Autodesk Fusion 360 part; units mm, degrees
sketch "Back Panel" plane through (0, 0, 0) normal (1, 0, 0) x (0, 1, 0)
  line L0 (0, 0) -> (6, 0)
  line L1 (6, 0) -> (6, 500.8)
  line L2 (0, 500.8) -> (0, 0)
  line L3 (0, 500.8) -> (0, 503.263)
  line L4 (6, 500.8) -> (0, 503.263)
  dimension "d8" = 6
  dimension "d9" = 500.8
  dimension "d10" = 2.463
  dimension "d11" = 112.318
extrude "Extrude2" add sketch "Back Panel" along normal blind 270
sketch "Switch Hole" plane through (0, 6, 0) normal (0, 1, 0) x (-1, 0, 0)
  line L0 (0, 0) -> (0, 500.8)
  line L1 (0, 500.8) -> (-270, 500.8)
  line L2 (-270, 500.8) -> (-270, 0)
  line L3 (-270, 0) -> (0, 0)
  line L4 (-234, 37) -> (-215, 37)
  line L5 (-215, 37) -> (-215, 24)
  line L6 (-215, 24) -> (-234, 24)
  line L7 (-234, 24) -> (-234, 37)
  dimension "d14" = 19
  dimension "d15" = 13
  dimension "d16" = 36
  dimension "d17" = 24
extrude "Extrude3" cut sketch "Switch Hole" against normal blind 6 contours L4 L5 L6 L7
sketch "Bottom Access Panel" plane through (0, 6, 0) normal (0, 1, 0) x (-1, 0, 0)
  line L0 (-215, 37) -> (-215, 24)
  line L1 (-215, 24) -> (-234, 24)
  line L2 (-234, 24) -> (-234, 37)
  line L3 (-234, 37) -> (-215, 37)
  line L4 (0, 0) -> (0, 500.8)
  line L5 (0, 500.8) -> (-270, 500.8)
  line L6 (-270, 500.8) -> (-270, 0)
  line L7 (-270, 0) -> (0, 0)
  line L8 (-205, 188) -> (-65, 188)
  line L9 (-65, 188) -> (-65, 48)
  line L10 (-65, 48) -> (-205, 48)
  line L11 (-205, 48) -> (-205, 188)
  dimension "d20" = 48
  dimension "d21" = 65
  dimension "d22" = 65
  dimension "d28" = 140
  dimension "d29" = 140
  dimension "d30" = 24
  dimension "d31" = 11
  dimension "d32" = 13
  dimension "d33" = 188
extrude "Extrude4" cut sketch "Bottom Access Panel" against normal blind 6 contours L8 L9 L10 L11
fillet "Fillet1" radius 8 4 edges at (65, 3, 188) (65, 3, 48) (205, 3, 48) (205, 3, 188)
sketch "Top Access Panel" plane through (0, 6, 0) normal (0, 1, 0) x (-1, 0, 0)
  line L0 (-65, 180) -> (-65, 56)
  arc A0 (-73, 48) -> (-65, 56) centre (-73, 56) ccw
  line L1 (-73, 48) -> (-197, 48)
  arc A1 (-205, 56) -> (-197, 48) centre (-197, 56) ccw
  line L2 (-205, 56) -> (-205, 180)
  arc A2 (-197, 188) -> (-205, 180) centre (-197, 180) ccw
  line L3 (-197, 188) -> (-73, 188)
  arc A3 (-65, 180) -> (-73, 188) centre (-73, 180) ccw
  line L4 (-215, 37) -> (-215, 24)
  line L5 (-215, 24) -> (-234, 24)
  line L6 (-234, 24) -> (-234, 37)
  line L7 (-234, 37) -> (-215, 37)
  line L8 (0, 0) -> (0, 500.8)
  line L9 (0, 500.8) -> (-270, 500.8)
  line L10 (-270, 500.8) -> (-270, 0)
  line L11 (-270, 0) -> (0, 0)
  line L12 (-195, 473.263) -> (-75, 473.263)
  line L13 (-75, 473.263) -> (-75, 383.263)
  line L14 (-75, 383.263) -> (-195, 383.263)
  line L15 (-195, 383.263) -> (-195, 473.263)
  line L16 (-180, 473.263) -> (-90, 473.263)
  line L17 (0, 503.263) -> (-270, 503.263)
  dimension "d34" = 120
  dimension "d35" = 140
  dimension "d36" = 75
  dimension "d37" = 75
  dimension "d38" = 65
  dimension "d39" = 65
  dimension "d45" = 90
  dimension "d49" = 30
extrude "Extrude5" cut sketch "Top Access Panel" against normal blind 6 contours L12 L13 L14 L15 L16
fillet "Fillet2" radius 8 4 edges at (75, 3, 473.263) (195, 3, 473.263) (195, 3, 383.263) (75, 3, 383.263)
equation "MDFThickness = 6 mm"
equation "d16 = ( 18 * 2 ) * 1 mm"
equation "d17 = ( 12 * 2 ) * 1 mm"
equation "filletRadius = 8 mm"
equation "d27 = filletRadius"
equation "d36 = ( ( 270 - 120 ) / 2 ) * 1 mm"
equation "d54 = filletRadius"
CAD build for the part. Positions are in the model's coordinates, mm. Round coordinates to 2 decimals unless told otherwise and drop trailing zeros. Loops run counter-clockwise (first coordinate to the right, second up) from the corner with the lowest first, then second, coordinate; pieces in that order, holes last. Notation, with made-up numbers: M -5.75,71.25 L 29.25,71.25 A22 cw 29.25,99.25 Z; hole C 1,86.5 d11. An arc over 180 degrees is marked long. One line per question, with ' | ' between items. Start each with the question number.
Item 1: Cut at B-B, the plane z = 115.5. Write the cut outline in (x, y).
Item 2: Cut at C-C, the plane y = 1.25. Write the cut outline in (x, z).
Item 3: Cut at D-D, the plane z = 422. Write the cut outline in (x, y), plus the area to 3 significant figures.
Item 4: Wall check: line 1 (Z direction, x = 168, y = 2.35); line 2 (Z direction, x = 76, y = 4.1); line 3 (X direction, y = 2.45, z = 61.5). Give the ranges that are in metal, low to high.
Item 5: Pin check, flat tips, straight feed: pin 1 Ø1.8 at (x, y) = (220.5, 2.5) entering from +Z; pin 2 Ø3 at (x, y) = (142, 2) entering from +Z. Stop position of each tip, or through.
Item 6: Cut at A-A, the plane x = 136.5. Write the cut outline in (y, z).
Responses:
1) outline: M 0,0 L 65,0 L 65,6 L 0,6 Z; M 205,0 L 270,0 L 270,6 L 205,6 Z
2) outline: M 0,0 L 270,0 L 270,502.75 L 0,502.75 Z; hole M 65,56 A8 ccw 73,48 L 197,48 A8 ccw 205,56 L 205,180 A8 ccw 197,188 L 73,188 A8 ccw 65,180 Z; hole M 75,391.26 A8 ccw 83,383.26 L 187,383.26 A8 ccw 195,391.26 L 195,465.26 A8 ccw 187,473.26 L 83,473.26 A8 ccw 75,465.26 Z; hole M 215,24 L 234,24 L 234,37 L 215,37 Z
3) outline: M 0,0 L 75,0 L 75,6 L 0,6 Z; M 195,0 L 270,0 L 270,6 L 195,6 Z | area: 900 mm²
4) line 1: z = 0 to 48, 188 to 383.26, 473.26 to 502.3 | line 2: z = 0 to 48, 188 to 387.39, 469.14 to 501.58 | line 3: x = 0 to 65, 205 to 270
5) pin 1: stops at z = 502.61 | pin 2: stops at z = 503.06
6) outline: M 0,0 L 6,0 L 6,48 L 0,48 Z; M 0,188 L 6,188 L 6,383.26 L 0,383.26 Z; M 0,473.26 L 6,473.26 L 6,500.8 L 0,503.26 Z
